Here's how the part is built. I have some questions about the finished solid (model axes, mm). Round coordinates to 2 decimals unless told otherwise and drop trailing zeros. Order: outer loops, then holes, each group sorted by start corner. A loop starts at its lowest first (then second) coordinate and runs counter-clockwise, first axis right, second up. Notation, with made-up numbers: M 62,31.25 L 96,31.25 A31 ccw 96,64.25 Z; hole C -20.5,31.25 d9. An arc over 180 degrees is marked long. Write item = value, one per line. Start each with the question number.
Item 1: I want a section at B-B, the plane x = 0. List the corners of the cut face in (y, z) for me, plus the area to 3 significant figures.
Item 2: I'm going to push a flat-ended pin straight in: P1, Ø2.5, axis at x = 0, y = 20, coming from the +Z side. Where does the tip first touch, or does it pass through?
Item 3: I want a section at C-C, the plane z = 0.6. List the corners of the cut face in (x, y) for me.
Item 4: I want a section at A-A, the plane y = 0. List the corners of the cut face in (x, z) for me, plus the area to 3 significant figures.
Item 5: Please list where these lines run through material, in increasing order: L1, parallel to Y at x = 0, z = 1.25; L2, parallel to X at y = 170, z = 1.15; L3, parallel to Y at x = 5.75, z = 1.9.
```python
from build123d import *

# Parameters (mm, degrees)
SKETCH_1_R      = 2.1
EXTRUDE_1_DEPTH = 2


with BuildPart() as part:
    # Эскиз1 → Бобышка-Вытянуть1 (new body)
    with BuildSketch(Plane.XY):
        with BuildLine():
            Line((-7.5, 173), (-7.5, -3))
            ThreePointArc((-7.5, -3), (-6.914213562, -4.414213562), (-5.5, -5))
            Line((-5.5, -5), (5.5, -5))
            ThreePointArc((5.5, -5), (6.914213562, -4.414213562), (7.5, -3))
            Line((7.5, -3), (7.5, 173))
            ThreePointArc((7.5, 173), (6.914213562, 174.414213562), (5.5, 175))
            Line((5.5, 175), (-5.5, 175))
            ThreePointArc((-5.5, 175), (-6.914213562, 174.414213562), (-7.5, 173))
        make_face()
        with Locations((0, 170)):
            Circle(SKETCH_1_R, mode=Mode.SUBTRACT)
        with Locations((0, 150)):
            Circle(SKETCH_1_R, mode=Mode.SUBTRACT)
        with Locations((0, 20)):
            Circle(SKETCH_1_R, mode=Mode.SUBTRACT)
        Circle(SKETCH_1_R, mode=Mode.SUBTRACT)
    extrude(amount=EXTRUDE_1_DEPTH)


solid = part.part
```
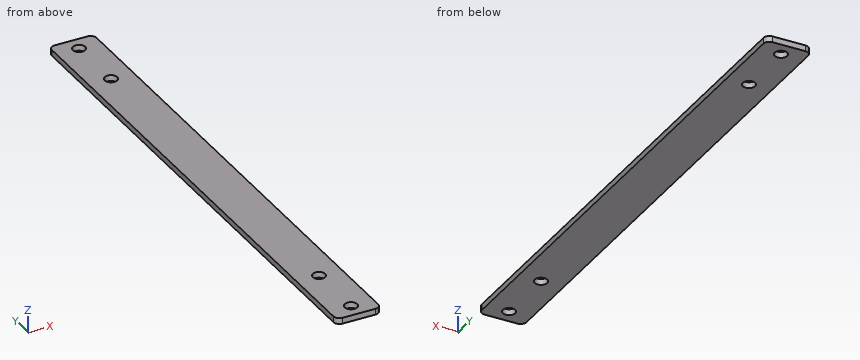
Filled in:
q1.outline = M -5,0 L -2.1,0 L -2.1,2 L -5,2 Z; M 2.1,0 L 17.9,0 L 17.9,2 L 2.1,2 Z; M 22.1,0 L 147.9,0 L 147.9,2 L 22.1,2 Z; M 152.1,0 L 167.9,0 L 167.9,2 L 152.1,2 Z; M 172.1,0 L 175,0 L 175,2 L 172.1,2 Z
q1.area = 326 mm^2
q2.P1 = through
q3.outline = M -7.5,-3 A2 ccw -5.5,-5 L 5.5,-5 A2 ccw 7.5,-3 L 7.5,173 A2 ccw 5.5,175 L -5.5,175 A2 ccw -7.5,173 Z; hole C 0,0 d4.2; hole C 0,20 d4.2; hole C 0,150 d4.2; hole C 0,170 d4.2
q4.outline = M -7.5,0 L -2.1,0 L -2.1,2 L -7.5,2 Z; M 2.1,0 L 7.5,0 L 7.5,2 L 2.1,2 Z
q4.area = 21.6 mm^2
q5.L1 = -5 to -2.1, 2.1 to 17.9, 22.1 to 147.9, 152.1 to 167.9, 172.1 to 175
q5.L2 = -7.5 to -2.1, 2.1 to 7.5
q5.L3 = -4.98 to 174.98
